CAD build for the part. Positions are in the model's coordinates, mm. A direction names the side the tool comes from. Round coordinates to 2 decimals unless told otherwise and drop trailing zeros. Write each loop counter-clockwise with the first axis right and the second up, starting at its lowest first coordinate (ties: lowest second). Pieces come first, ordered by that corner, then holes. Notation, with made-up numbers: (31, 25.25) - (35, 25.25) arc R31 cw to (35, 64.25) - close; hole circle Ø3 at (40, -30). An arc over 180 degrees is marked (long way). Put each result on its own line as item: value. Start each with the question number.
Item 1: Cut at B-B (y = 7). Give the cut face in (x, z), and give its area (3 significant figures).
Item 2: 3-axis set-ups, long thin cutter, end or side, ignore diameter. For faces 5 (the flat face through (-19, 6, 2.2)), 6 (the flat face through (-22, 13, 4.5)): which of +Z, -Z, +X, -X, +Y, -Y reach the whole face in a straight line?
Item 3: Drill centre lines: line 1 (Y direction, x = -32, z = 0.55); line 2 (X direction, y = 10, z = 3); line 3 (Z direction, x = -15, y = 2.5). Where is each one in solid material? Low to high. Write a range as from..to.
Item 4: Cut at A-A (x = -32). Give the cut face in (y, z).
Item 5: Mould opens along X. For faces 1 (the flat face through (0, 7, 2)), 2 (the flat face through (-38.3, 8, 2)), 3 (the cylindrical face through (-3.44, 7.9, 1.08)), 4 (the flat face through (-19, 15, 2)) say: released by +X, released by -X, zero draft, split by the parting line, or undercut.
Item 6: Pin check, flat tips, straight feed: pin 1 Ø7 at (x, y) = (-6.3, 7) entering from -Z; pin 2 Ø0.7 at (x, z) = (-15.5, 3.5) entering from -Y. Stop position of each tip, or through.
Item 7: Cut at D-D (z = 3.25). Give the cut face in (x, y).
Item 8: Cut at C-C (z = 0.4). Give the cut face in (x, y), and give its area (3 significant figures).
```python
from build123d import *

# Parameters (mm, degrees)
F0_W     = 38.3
F0_H     = 15
F0_R     = 3
F1_DEPTH = 2.2
F3_DEPTH = 2.3


with BuildPart() as f1:
    # F0 (on Top) → F1 (new body)
    with BuildSketch(Plane.XY):
        with Locations((-19.15, 7.5)):
            Rectangle(F0_W, F0_H)
        with Locations((-32, 7)):
            Circle(F0_R, mode=Mode.SUBTRACT)
        with Locations((-6.3, 7)):
            Circle(F0_R, mode=Mode.SUBTRACT)
    extrude(amount=F1_DEPTH)

    # F2 (on face) → F3 (join)
    with BuildSketch(Plane.XY.offset(2.2)):
        Polygon((0, 15), (-38.3, 15), (-38.3, 0), (-36.1, 0), (-36.1, 12.8), (-2.2, 12.8), (-2.2, 0), (0, 0), align=None)
    extrude(amount=F3_DEPTH)


solid = f1.part
```
Output values:
1. outline: (-38.3, 0) - (-35, 0) - (-35, 2.2) - (-36.1, 2.2) - (-36.1, 4.5) - (-38.3, 4.5) - close; (-29, 0) - (-9.3, 0) - (-9.3, 2.2) - (-29, 2.2) - close; (-3.3, 0) - (0, 0) - (0, 4.5) - (-2.2, 4.5) - (-2.2, 2.2) - (-3.3, 2.2) - close
1. area: 68.0 mm2
2. face 5: +Z, -Y
2. face 6: +Z, +X, -X, +Y, -Y
3. line 1: 0..4, 10..15
3. line 2: -38.3..-36.1, -2.2..0
3. line 3: 0..2.2
4. outline: (0, 0) - (4, 0) - (4, 2.2) - (0, 2.2) - close; (10, 0) - (15, 0) - (15, 4.5) - (12.8, 4.5) - (12.8, 2.2) - (10, 2.2) - close
5. face 1: released by +X
5. face 2: released by -X
5. face 3: undercut
5. face 4: zero draft
6. pin 1: z = 0
6. pin 2: y = 12.8
7. outline: (-38.3, 0) - (-36.1, 0) - (-36.1, 12.8) - (-2.2, 12.8) - (-2.2, 0) - (0, 0) - (0, 15) - (-38.3, 15) - close
8. outline: (-38.3, 0) - (0, 0) - (0, 15) - (-38.3, 15) - close; hole circle Ø6 at (-32, 7); hole circle Ø6 at (-6.3, 7)
8. area: 518 mm2
